Can you work these out from the model? Positions are in its coordinate system, mm. A direction names the side the tool comes from. Round coordinates to 2 decimals unless told otherwise and drop trailing zeros. Order: outer loops, then holes, each group sorted by start corner. A loop starts at its lowest first (then second) coordinate and runs counter-clockwise, first axis right, second up. Notation, with made-up numbers: (55.25, -26.5) -> (71.25, -26.5) arc R19 ccw to (71.25, 6.5) -> close; hole circle Ø1 at (-9.75, 23). An arc over 180 degrees is marked (long way). Use a Markdown table: item, result. Add a question column.
Q1. I need wall thicknesses on line 1 along X through (y, z) = (46, 2.25); line 2 along Y through (x, z) = (-188.5, 28). Which ranges of each line are inside material? Lowest first, please. Write a range as [from, to].
Q2. If we section it at B-B on x = 42.5: List the corners of the cut face in (y, z) for me.
Q3. If we section it at A-A on y = 49: List the corners of the cut face in (x, z) for me.
Q4. If we section it at C-C on z = 24.5: List the corners of the cut face in (x, y) for me.
Q5. I'm going to push flat-ended pins straight in: pin 1 Ø2.5 at (x, z) = (-502, 2) entering from +Y; pin 2 Ø5 at (x, z) = (-408, 23) entering from +Y; pin 3 Ø10 at (x, z) = (-246, 8.5) entering from +Y; pin 4 Ø4 at (x, y) = (-562, 28.5) entering from +Z. Where does each tip first touch, or does it pass through?
Q6. For faces 1 (the face through (10, 3, 18)), 2 (the face through (750, 24.3, 2.8)), which set-ups out of +Z, -Z, +X, -X, +Y, -Y let a thin tool reach every point of the face, with its end or its side?
Autodesk Inventor part; units mm, degrees
ref_plane "YZ Plane" through (0, 0, 0) normal (1, 0, 0) x (0, 1, 0)
ref_plane "XZ Plane" through (0, 0, 0) normal (0, 1, 0) x (-1, 0, 0)
ref_plane "XY Plane" through (0, 0, 0) normal (0, 0, 1) x (1, 0, 0)
sketch "Sketch1" plane through (0, 0, 0) normal (0, 0, 1) x (1, 0, 0)
  line L0 (-750, 77.9594) -> (750, 77.9594)
  line L1 (750, 77.9594) -> (750, 0)
  line L2 (750, 0) -> (-750, 0)
  line L3 (-750, 0) -> (-750, 77.9594)
  point P0 (0, 0)
  point P1 (0, 0)
  dimension "d0" = 1500
  dimension "d1" = 77.9594
extrude "Plate1" add sketch "Sketch1" along normal blind 3
sketch "Sketch2" plane through (750, 3, 0) normal (0, -1, 0) x (1, 0, 0)
  line L0 (-1500, 0) -> (0, 0)
  line L1 (0, 0) -> (0, 30)
  line L2 (0, 30) -> (-1500, 30)
  line L3 (-1500, 30) -> (-1500, 0)
edge flange "Flange1" height 30 angle 90 thickness 3 bend radius 3 thickness toward (0, -1, 0) relief tear relief width 3 relief depth 1.5 edges at (0, 0, 3) wall of the first edge with corners at (-750, 3, 0) (750, 3, 0) (750, 3, 30) (-750, 3, 30)
bend "Bend1"
corner "Corner1"
sketch "Sketch5" plane through (0, 0, 0) normal (0, 0, -1) x (-1, 0, 0)
  line L0 (750, 77.9594) -> (-750, 77.9594)
  line L1 (500, 77.9594) -> (500, 31)
  line L2 (500, 31) -> (503, 31)
  line L3 (503, 31) -> (503, 77.9594)
  line L4 (750, 0) -> (-750, 0)
  point P0 (0, 0)
  dimension "d18" = 3
  dimension "d19" = 247
  dimension "d20" = 31
extrude "Extrusion1" cut sketch "Sketch5" against normal through all
pattern_linear "Rectangular Pattern1" count 3 spacing 500 along (1, 0, 0) of "Extrusion1"
sketch "Sketch6" plane through (0, 0, 0) normal (0, 0, -1) x (-1, 0, 0)
  line L0 (-750, 77.9594) -> (-750, 6)
  circle A0 centre (-750, 77.9594) radius 15
  line L1 (-750, 77.9594) -> (-500, 77.9594)
  point P0 (0, 0)
  point P1 (-735, 77.9594)
  point P2 (-750, 62.9594)
  dimension "d24" = 30
extrude "Extrusion2" cut sketch "Sketch6" against normal through all contours L1 A0 L0 picked at (-740.1254, 76.8468)
mirror "Mirror1" about plane through (0, 0, 0) normal (1, 0, 0) of "Extrusion2"
equation "\"d1\" = Стрингер_6"
equation "\"d18\" = Thickness"
equation "\"d2\" = Thickness"
equation "\"d3\" = BendReliefWidth"
equation "\"d4\" = BendReliefDepth"
equation "\"d5\" = MinimumRemnant"
equation "\"d6\" = TransitionRadius"
equation "\"d9\" = BendRadius"
equation "\"d10\" = CornerReliefSize"
equation "\"d11\" = GapSize"
equation "\"d12\" = JacobiRadiusSize"
equation "\"BendRadius\" = Thickness"
equation "\"BendReliefWidth\" = Thickness"
equation "\"BendReliefDepth\" = 0.5 * Thickness"
equation "\"CornerReliefSize\" = 4 * Thickness"
equation "\"MinimumRemnant\" = 2 * Thickness"
equation "\"TransitionRadius\" = BendRadius"
equation "\"JacobiRadiusSize\" = BendRadius"
equation "\"GapSize\" = Thickness"
properties part number "МОО 056 стрингер борт 6"
Answer below:
| question | item | result |
|---|---|---|
| 1 | line 1 | [-750, -503], [-500, -3], [0, 497], [500, 750] |
| 1 | line 2 | [0, 3] |
| 2 | outline | (0, 6) arc R6 ccw to (6, 0) -> (77.96, 0) -> (77.96, 3) -> (6, 3) arc R3 cw to (3, 6) -> (3, 30) -> (0, 30) -> close |
| 3 | outline | (-750, 0) -> (-503, 0) -> (-503, 3) -> (-750, 3) -> close; (-500, 0) -> (-3, 0) -> (-3, 3) -> (-500, 3) -> close; (0, 0) -> (497, 0) -> (497, 3) -> (0, 3) -> close; (500, 0) -> (750, 0) -> (750, 3) -> (500, 3) -> close |
| 4 | outline | (-750, 0) -> (750, 0) -> (750, 3) -> (-750, 3) -> close |
| 5 | pin 1 | y = 77.96 |
| 5 | pin 2 | y = 3 |
| 5 | pin 3 | y = 4.34 |
| 5 | pin 4 | z = 3 |
| 6 | face 1 | +Z, +X, -X, +Y |
| 6 | face 2 | +Z, -Z, +X, +Y, -Y |
